For this review, take the finished solid that the model builds, in its own axes (mm). A direction names the side the tool comes from. Round coordinates to 2 decimals unless told otherwise and drop trailing zeros. Loops run counter-clockwise (first coordinate to the right, second up) from the corner with the lowest first, then second, coordinate; pieces in that order, holes last.
1. Draft analysis for pull direction Z (two halves, no side actions). For faces 4 (the flat face through (-52.22, 41.86, 29.14)), 5 (the cylindrical face through (31.188, 2.231, 25.737)), 6 (the flat face through (-26, 44.4, 54)), state which applies: released by +Z, released by -Z, zero draft, split by the parting line, or undercut.
2. To check wall thickness, follow line 1 along Z through (x, y) = (-0.5, 4); line 2 along Z through (x, y) = (-0.5, 16); line 3 along Y through (x, z) = (11.5, 53). State the ranges of each line that lie inside material, in increasing order.
3. Consider section C-C on z = 15.5. State the section outline as (x, y) points.
4. Clearance check with flat-ended pins moving along their axes: pin 1 Ø3.5 at (x, y) = (-7, 1.5) entering from +Z; pin 2 Ø23 at (x, y) = (21.5, 13) entering from -Z; pin 3 Ø23 at (x, y) = (28.5, 15.5) entering from +Z. State where each tip first meets the part, or that it passes through.
5. Consider section D-D on y = 14. State the section outline as (x, z) points.
6. Tool access review of faces 1 (the flat face through (35, 7, 40.2)), 2 (the flat face through (40.523, 2.175, -32.186)), 3 (the flat face through (-35.053, 41.935, 48.662)): name each direction out of +Z, -Z, +X, -X, +Y, -Y from which nothing blocks a thin tool from reaching the whole face with its end or side.
7. Consider section A-A on y = 34. State the section outline as (x, z) points.
8. Consider section B-B on x = 9. State the section outline as (y, z) points, then the cut area to 3 significant figures.
from build123d import *

# Parameters (mm, degrees)
BOSS_EXTRUDE1_DEPTH     = 4.4
BOSS_EXTRUDE2_START     = 4.4
BOSS_EXTRUDE2_DEPTH     = 40
BOSS_EXTRUDE3_START     = 4.4
BOSS_EXTRUDE3_DEPTH     = 3
CUT_EXTRUDE1_START      = -37
CUT_EXTRUDE1_DEPTH      = 37
CHAMFER1_SIZE           = 5
CUT_EXTRUDE2_DEPTH      = 120.718001988
CUT_EXTRUDE2_DEPTH_BACK = 120.718001988
FILLET1_R               = 10
CUT_EXTRUDE3_START      = -15
CUT_EXTRUDE3_DEPTH      = 80.4


with BuildPart() as part:
    # Sketch1 → Boss-Extrude1 (new body)
    with BuildSketch(Plane(origin=(0, 0, 0), x_dir=(1, 0, 0), z_dir=(0, 1, 0))):
        with BuildLine():
            Line((-31.320919527, 25.2), (31.320919527, 25.2))
            Line((31.320919527, 25.2), (51.0779796, 40.2))
            ThreePointArc((51.0779796, 40.2), (-65, 0), (51.0779796, -40.2))
            Line((51.0779796, -40.2), (31.320919527, -25.2))
            Line((31.320919527, -25.2), (-31.320919527, -25.2))
            ThreePointArc((-31.320919527, -25.2), (-40.2, 0), (-31.320919527, 25.2))
        make_face()
    extrude(amount=BOSS_EXTRUDE1_DEPTH)

    # Sketch1<3> → Boss-Extrude2 (add)
    with BuildSketch(Plane(origin=(0, 0, 0), x_dir=(1, 0, 0), z_dir=(0, 1, 0)).offset(BOSS_EXTRUDE2_START)):
        with BuildLine():
            ThreePointArc((37.536115942, -40.2), (-21.914762413, -50.445447648), (-55, 0))
            Line((-55, 0), (-65, 0))
            ThreePointArc((-65, 0), (-21.271240279, -61.420960079), (51.0779796, -40.2))
            Line((51.0779796, -40.2), (37.536115942, -40.2))
        make_face()
        with BuildLine():
            ThreePointArc((-55, 0), (-21.914762413, 50.445447648), (37.536115942, 40.2))
            Line((37.536115942, 40.2), (51.0779796, 40.2))
            ThreePointArc((51.0779796, 40.2), (-21.271240279, 61.420960079), (-65, 0))
            Line((-65, 0), (-55, 0))
        make_face()
    extrude(amount=BOSS_EXTRUDE2_DEPTH)

    # Sketch1<4> → Boss-Extrude3 (add)
    with BuildSketch(Plane(origin=(0, 0, 0), x_dir=(1, 0, 0), z_dir=(0, 1, 0)).offset(BOSS_EXTRUDE3_START)):
        with BuildLine():
            ThreePointArc((-40.2, 0), (-37.915306704, 13.359248389), (-31.320919527, 25.2))
            ThreePointArc((-31.320919527, 25.2), (-17.363755354, 36.256585609), (0, 40.2))
            Line((0, 40.2), (37.536115942, 40.2))
            ThreePointArc((37.536115942, 40.2), (-21.914762413, 50.445447648), (-55, 0))
            Line((-55, 0), (-40.2, 0))
        make_face()
        with BuildLine():
            ThreePointArc((-31.320919527, -25.2), (-37.915306704, -13.359248389), (-40.2, 0))
            Line((-40.2, 0), (-55, 0))
            ThreePointArc((-55, 0), (-21.914762413, -50.445447648), (37.536115942, -40.2))
            Line((37.536115942, -40.2), (0, -40.2))
            ThreePointArc((0, -40.2), (-17.363755354, -36.256585609), (-31.320919527, -25.2))
        make_face()
    extrude(amount=BOSS_EXTRUDE3_DEPTH)

    # Sketch2 → Cut-Extrude1 (cut)
    with BuildSketch(Plane(origin=(0, 44.4, 0), x_dir=(1, 0, 0), z_dir=(0, 1, 0)).offset(CUT_EXTRUDE1_START)):
        with BuildLine():
            Line((-47.304535151, -28.058527299), (-54.891163788, -34.813217864))
            ThreePointArc((-54.891163788, -34.813217864), (-48.54657249, -43.223029736), (-40.926800335, -50.49749513))
            Line((-40.926800335, -50.49749513), (-33.340171698, -43.742804564))
            ThreePointArc((-33.340171698, -43.742804564), (-41.07786903, -36.573332853), (-47.304535151, -28.058527299))
        make_face()
    extrude(amount=CUT_EXTRUDE1_DEPTH, mode=Mode.SUBTRACT)

    # Chamfer1
    chamfer1_edges = [part.edges().sort_by_distance(p)[0] for p in [
        (-51.097849469, 44.4, 31.435872581),
        (-37.133486016, 44.4, 47.120149847),
    ]]
    chamfer(chamfer1_edges, length=CHAMFER1_SIZE)

    # Sketch3 → Cut-Extrude2 (cut, two sides: drawn at the far end of the back side and taken through both)
    with BuildSketch(Plane.XY.offset(-25.2).offset(-CUT_EXTRUDE2_DEPTH_BACK)):
        with BuildLine():
            Line((51.0779796, 44.4), (-18.9220204, 44.4))
            ThreePointArc((-18.9220204, 44.4), (20.209169206, 35.162379212), (51.0779796, 9.4))
            Line((51.0779796, 9.4), (51.0779796, 44.4))
        make_face()
    extrude(amount=CUT_EXTRUDE2_DEPTH + CUT_EXTRUDE2_DEPTH_BACK, mode=Mode.SUBTRACT)

    # Fillet1
    fillet1_edges = [part.edges().sort_by_distance(p)[0] for p in [
        (31.320919527, 2.2, -25.2),
        (31.320919527, 2.2, 25.2),
    ]]
    fillet(fillet1_edges, radius=FILLET1_R)

    # Sketch4 → Cut-Extrude3 (cut)
    with BuildSketch(Plane.XY.offset(-25.2).offset(CUT_EXTRUDE3_START)):
        Polygon((51.0779796, 4.4), (27.954908691, 4.4), (51.0779796, 2.9), align=None)
        Polygon((51.0779796, 0), (51.0779796, 1.5), (27.954908691, 0), align=None)
    extrude(amount=CUT_EXTRUDE3_DEPTH, mode=Mode.SUBTRACT)


solid = part.part
Resolved:
1. face 4: released by +Z
1. face 5: undercut
1. face 6: zero draft
2. line 1: z = -65 to -25.2, 25.2 to 65
2. line 2: z = -65 to -55, 55 to 65
2. line 3: y = 0 to 7.4
3. outline: (-63.12, 0) - (-37.09, 0) - (-37.09, 7.4) - (-52.77, 7.4) - (-52.77, 44.4) - (-63.12, 44.4) - close
4. pin 1: stops at z = 64.79
4. pin 2: stops at z = -64.23
4. pin 3: stops at z = 62.74
5. outline: (-54.89, 34.81) arc R65 ccw to (47.38, -44.5) - (47.38, -40.2) - (37.54, -40.2) arc R55 cw to (-47.3, 28.06) - close; (-40.93, 50.5) - (-33.34, 43.74) arc R55 cw to (37.54, 40.2) - (47.38, 40.2) - (47.38, 44.5) arc R65 ccw to start
6. face 1: +X, +Y
6. face 2: +X, +Y, -Y
6. face 3: -X, +Y
7. outline: (-54.89, 34.81) arc R65 ccw to (22.45, -61) - (22.45, -50.21) arc R55 cw to (-47.3, 28.06) - close; (-40.93, 50.5) - (-33.34, 43.74) arc R55 cw to (22.45, 50.21) - (22.45, 61) arc R65 ccw to start
8. outline: (0, -64.37) - (39.83, -64.37) - (39.83, -54.26) - (7.4, -54.26) - (7.4, -40.2) - (4.4, -40.2) - (4.4, -25.2) - (0, -25.2) - close; (0, 25.2) - (4.4, 25.2) - (4.4, 40.2) - (7.4, 40.2) - (7.4, 54.26) - (39.83, 54.26) - (39.83, 64.37) - (0, 64.37) - close
8. area: 1,150 mm2
